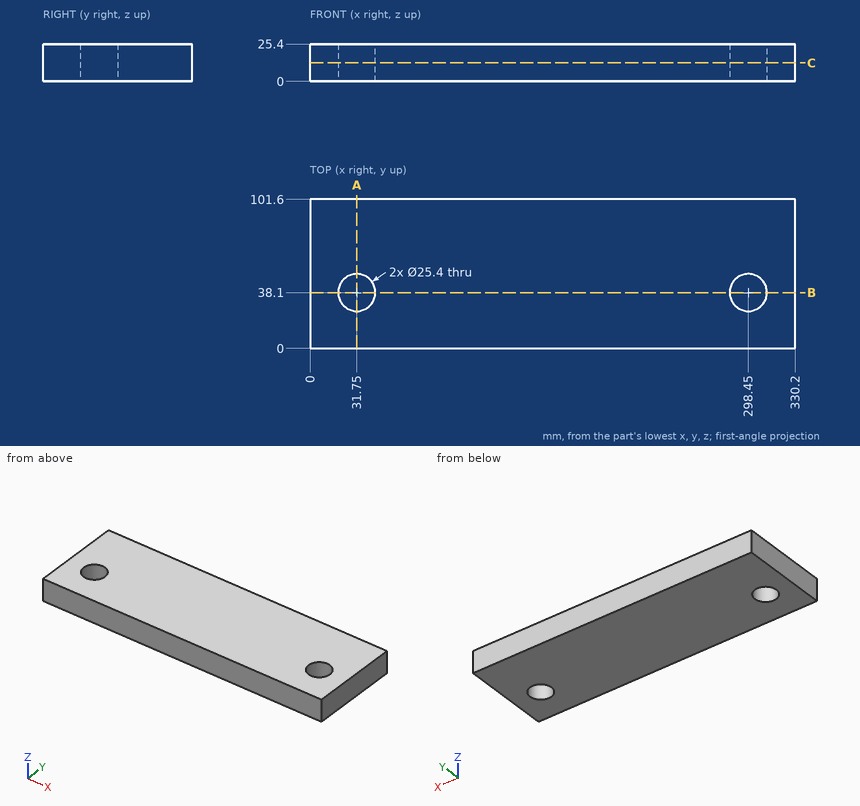
Answer from the drawing. Dimensions are ordinates in mm from the lowest x, y and z of the part. Give positions to 0.01 mm unless a question says otherwise; leave off trailing zeros. Write each loop counter-clockwise with the first axis right and the second up, starting at its lowest first coordinate (ties: lowest second). Pieces come first, ordered by that corner, then holes. Notation, with made-up numbers: (60.25, 4) - (77.25, 4) arc R20 cw to (77.25, 26) - close; hole circle Ø4 at (20, 38). An arc over 180 degrees is marked (long way). One line per item, written item: value. Start each with the question number.
1. Find section B-B (y = 38.1). Write down the section's boundary in (x, z), then the cut area to 3 significant figures.
2. Find section C-C (z = 12.5). Write down the section's boundary in (x, y), then the cut area to 3 significant figures.
3. Find section A-A (x = 31.75). Write down the section's boundary in (y, z).
4. Given pin 1 (4 mm diameter, centred on x = 173.5, z = 8.5, fed in from -Y); pin 2 (20.5 mm diameter, centred on x = 31.75, y = 38.1, fed in from +Z), each flat-ended and moving along its own axis, determine where each tip first touches the part or whether it passes through.
5. Consider probe 1 along Y at (x, z) = (298.45, 16.5); probe 2 along X at (y, z) = (33, 16.25); probe 3 along X at (y, z) = (31.5, 20.25). Determine where each line is inside the solid, lowest interval first.
Geometry results:
1. outline: (0, 0) - (19.05, 0) - (19.05, 25.4) - (0, 25.4) - close; (44.45, 0) - (285.75, 0) - (285.75, 25.4) - (44.45, 25.4) - close; (311.15, 0) - (330.2, 0) - (330.2, 25.4) - (311.15, 25.4) - close
1. area: 7,100 mm2
2. outline: (0, 0) - (330.2, 0) - (330.2, 101.6) - (0, 101.6) - close; hole circle Ø25.4 at (31.75, 38.1); hole circle Ø25.4 at (298.45, 38.1)
2. area: 32,500 mm2
3. outline: (0, 0) - (25.4, 0) - (25.4, 25.4) - (0, 25.4) - close; (50.8, 0) - (101.6, 0) - (101.6, 25.4) - (50.8, 25.4) - close
4. pin 1: y = 0
4. pin 2: through
5. probe 1: 0 to 25.4, 50.8 to 101.6
5. probe 2: 0 to 20.12, 43.38 to 286.82, 310.08 to 330.2
5. probe 3: 0 to 20.9, 42.6 to 287.6, 309.3 to 330.2
